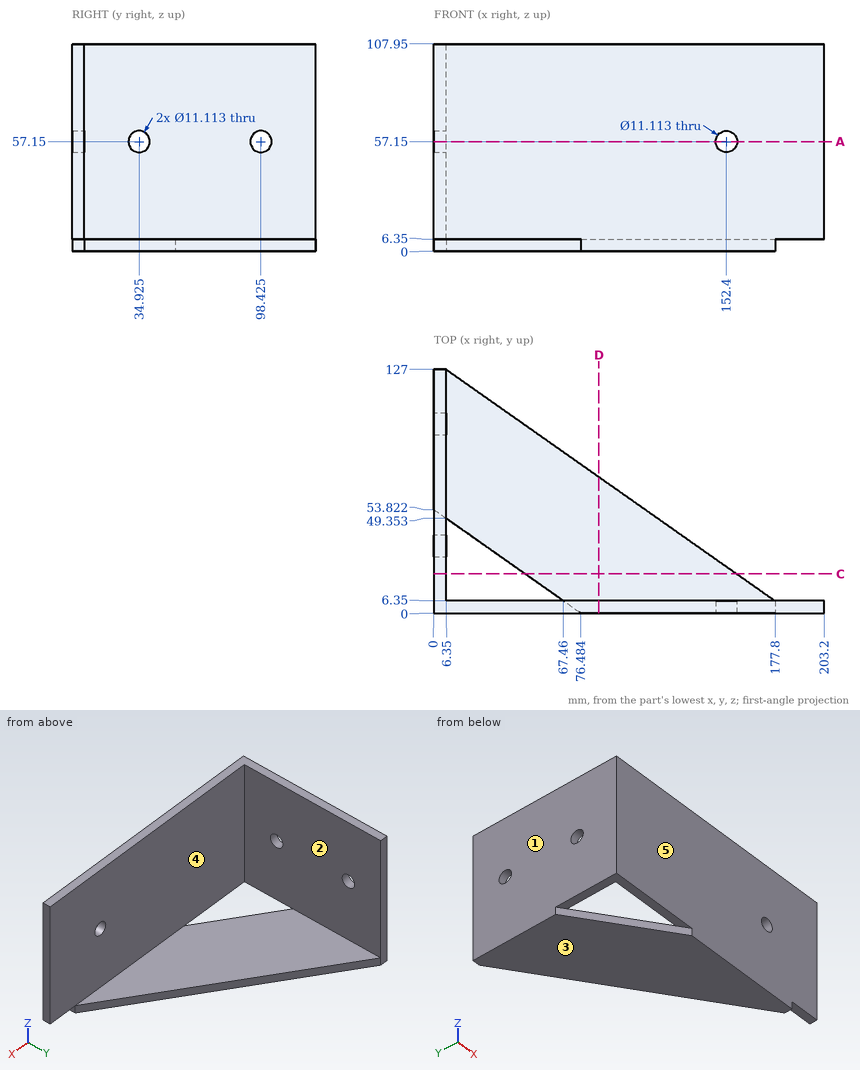
Geometry check sheet. Reference: drawing and pictorial views, mm from the part's lowest x, y, z. A direction names the side the tool comes from. Round coordinates to 2 decimals unless told otherwise and drop trailing zeros. Order: outer loops, then holes, each group sorted by start corner. A loop starts at its lowest first (then second) coordinate and runs counter-clockwise, first axis right, second up. Notation, with made-up numbers: M 75.5,59.5 L 106.5,59.5 A13 cw 106.5,82.5 Z; hole C 89.25,-40 d9. An arc over 180 degrees is marked long. Answer as CSV lines item,"result".
1) Thickness scan on probe 1 along X at (y, z) = (56, 78). Record the ranges inside material, lowest first. Write a range as [from, to].
Entries:
probe 1,"[0, 6.35]"
2) Sectioned sample at D-D on x = 86. Record the cut outline in (y, z), and give its area (3 significant figures).
Entries:
outline,"M 0,0 L 70.95,0 L 70.95,6.35 L 6.35,6.35 L 6.35,107.95 L 0,107.95 Z"
area,"1,100 mm2"
3) Sectioned sample at A-A on z = 57.15. Record the cut outline in (x, y).
Entries:
outline,"M 0,0 L 146.84,0 L 146.84,6.35 L 6.35,6.35 L 6.35,29.37 L 0,29.37 Z; M 0,40.48 L 6.35,40.48 L 6.35,92.87 L 0,92.87 Z; M 0,103.98 L 6.35,103.98 L 6.35,127 L 0,127 Z; M 157.96,0 L 203.2,0 L 203.2,6.35 L 157.96,6.35 Z"
4) Gauge pin test, flat ends, axial feed: pin 1 Ø5 at (x, y) = (185, 4) entering from -Z; pin 2 Ø2 at (x, z) = (161.5, 41.5) entering from +Y; pin 3 Ø5 at (y, z) = (4.5, 2) entering from +X; pin 4 Ø10 at (x, y) = (92, 78.5) entering from +Z (3 decimals). Record the tip position at first contact, or that the pin passes through.
Entries:
pin 1,"z = 6.35"
pin 2,"y = 6.35"
pin 3,"x = 177.8"
pin 4,"through"
5) Mould release check, pull along X, two halves, no side actions. Record for the marked faces 1, 2 and 3: +X half, -X half, draft (parallel to the pull), parting line (faces both ways), or undercut.
Entries:
face 1,"-X half"
face 2,"+X half"
face 3,"draft"
6) Tool access check on the marked faces 4 and 5. Record the directions out of +Z, -Z, +X, -X, +Y, -Y that give a thin tool (end or side, any length) a straight path to the whole face; none if there is none.
Entries:
face 4,"+Z, +X, +Y"
face 5,"+Z, -Z, +X, -X, -Y"
7) Sectioned sample at C-C on y = 20.5. Record the cut outline in (x, z).
Entries:
outline,"M 0,6.35 L 6.35,6.35 L 6.35,107.95 L 0,107.95 Z; M 47.35,0 L 157.69,0 L 157.69,6.35 L 47.35,6.35 Z"
